Could you check a few things on this model? Use its own coordinates, in mm. Face numbers are marked on the shaded views. A direction names the side the tool comes from. Give positions to 0.01 mm unless a question says otherwise; leave off trailing zeros. Loops run counter-clockwise (first coordinate to the right, second up) from the corner with the lowest first, then second, coordinate; pieces in that order, holes last. Notation, with made-up numbers: M 75.5,-23 L 132.5,-23 A21 cw 132.5,1 Z; hole C 66,0.5 d9. An arc over 180 degrees is marked long. Use CSV: the item, a comma, the result in double quotes.
```python
from build123d import *

# Parameters (mm, degrees)
BASPROSKE_W         = 5
BASPROSKE_H         = 12.75
TOOTHCUT_DEPTH      = 19.711627401
TEETHCUTS_COUNT     = 15
TEETHCUTS_ANGLE     = 336
BORSKE_R            = 2.7
BORE_DEPTH          = 50.0049784
SKETCH3_R           = 2.7
BOSS_EXTRUDE2_DEPTH = 5
FILLET1_R           = 5


with BuildPart() as part:
    # BasProSke → Base-Revolve (revolve)
    with BuildSketch(Plane(origin=(0, 0, 0), x_dir=(1, 0, 0), z_dir=(0, 1, 0)), mode=Mode.PRIVATE) as base_revolve_sk:
        with Locations((2.5, 6.375)):
            Rectangle(BASPROSKE_W, BASPROSKE_H)
    revolve(base_revolve_sk.sketch.rotate(Axis((-10, 0, 0), (1, 0, 0)), 180), axis=Axis((-10, 0, 0), (1, 0, 0)))

    # TooCutSke → ToothCut (cut, through all)
    with BuildSketch(Plane(origin=(0, 0, 0), x_dir=(0, 0, -1), z_dir=(1, 0, 0))):
        with BuildLine():
            ThreePointArc((0.769645606, 9.34235097), (0, 9.374), (-0.769645606, 9.34235097))
            ThreePointArc((-0.769645606, 9.34235097), (-1.209019537, 11.113083179), (-2.315283452, 12.563849239))
            ThreePointArc((-2.315283452, 12.563849239), (0, 12.7754), (2.315283452, 12.563849239))
            ThreePointArc((2.315283452, 12.563849239), (1.209019537, 11.113083179), (0.769645606, 9.34235097))
        make_face()
    toothcut = extrude(amount=TOOTHCUT_DEPTH, mode=Mode.SUBTRACT)

    # TeethCuts: ToothCut ×15 about axis
    teethcuts_axis = Axis((-10, 0, 0), (1, 0, 0))
    for i in range(1, TEETHCUTS_COUNT):
        add(toothcut.rotate(teethcuts_axis, i * TEETHCUTS_ANGLE / (TEETHCUTS_COUNT - 1)), mode=Mode.SUBTRACT)

    # BorSke → Bore (cut, symmetric)
    with BuildSketch(Plane(origin=(0, 0, 0), x_dir=(0, 0, -1), z_dir=(1, 0, 0))):
        with Locations(Location((0, 0, 0), (0, 0, 180))):
            Circle(BORSKE_R)
    extrude(amount=BORE_DEPTH, both=True, mode=Mode.SUBTRACT)

    # Sketch3 → Boss-Extrude2 (add)
    with BuildSketch(Plane.ZY):
        with BuildLine():
            Line((-5.518933108, -11.493645085), (-4, -18.283482979))
            Line((-4, -18.283482979), (-4, -50))
            ThreePointArc((-4, -50), (0, -54), (4, -50))
            Line((4, -50), (4, -18.283482979))
            Line((4, -18.283482979), (5.518933108, -11.493645085))
            Line((5.518933108, -11.493645085), (2.695210989, -8.978179867))
            Line((2.695210989, -8.978179867), (-2.695210989, -8.978179867))
            Line((-2.695210989, -8.978179867), (-5.518933108, -11.493645085))
        make_face()
        with Locations((0, -50)):
            Circle(SKETCH3_R, mode=Mode.SUBTRACT)
    extrude(amount=-BOSS_EXTRUDE2_DEPTH)

    # Fillet1
    fillet1_edges = [part.edges().sort_by_distance(p)[0] for p in [
        (2.5, -18.283482979, -4),
        (2.5, -18.283482979, 4),
    ]]
    fillet(fillet1_edges, radius=FILLET1_R)


solid = part.part
```
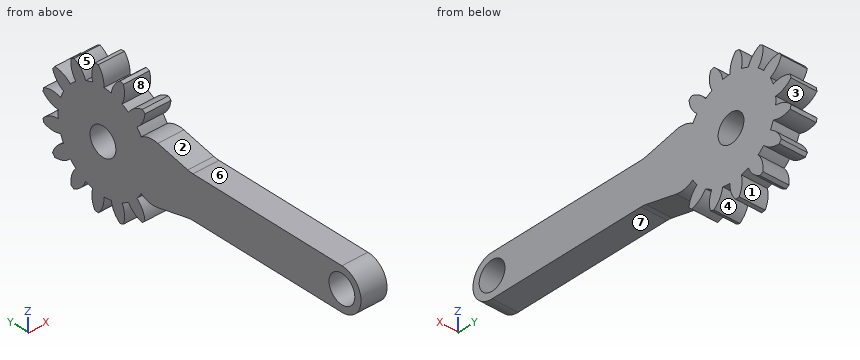
1. Which directions (+Z, -Z, +X, -X, +Y, -Y) give clear straight access to the entire face, cutting with the end or side of a thin tool? Please do the marked faces 4, 5, 6, 7 and 8.
Outcome:
face 4,"-Z, +X, -X"
face 5,"+Z, +X, -X"
face 6,"+Z, +X, -X, -Y"
face 7,"-Z, +X, -X, -Y"
face 8,"+X, -X"
2. I want a section at B-B, the plane x = 3.85. Give the number of separate pieces and of enclosed holes in the cut face, then the cut area to 3 significant figures.
Outcome:
separate pieces,"1"
enclosed holes,"2"
area,"686 mm2"
3. I want a section at C-C, the plane y = -34. List the corners of the cut face in (x, z) for me, then the cut area to 3 significant figures.
Outcome:
outline,"M 0,-4 L 5,-4 L 5,4 L 0,4 Z"
area,"40.0 mm2"
4. I want a section at A-A, the plane z = 0. List the corners of the cut face in (x, y) for me, then the cut area to 3 significant figures.
Outcome:
outline,"M 0,-54 L 5,-54 L 5,-52.7 L 0,-52.7 Z; M 0,-47.3 L 5,-47.3 L 5,-2.7 L 0,-2.7 Z; M 0,2.7 L 5,2.7 L 5,9.37 L 0,9.37 Z"
area,"263 mm2"
5. Please list where these lines run through material, in increasing order: line 1 (Y direction, x = 3.35, z = 0); line 2 (Z direction, x = 0.5, y = 9.5); line 3 (Z direction, x = 3.95, y = -27).
Outcome:
line 1,"-54 to -52.7, -47.3 to -2.7, 2.7 to 9.37"
line 2,"-7.75 to -5.45, -3.3 to -0.78, 0.78 to 3.3, 5.45 to 7.75"
line 3,"-4 to 4"
6. I'm going to push flat-ended pins straight in: pin 1 Ø1.5 at (x, y) = (2.5, -35.5) entering from +Z; pin 2 Ø4.5 at (y, z) = (-50, 0) entering from +X; pin 3 Ø12 at (y, z) = (-22.5, -7) entering from +X; pin 4 Ø1.5 at (x, z) = (4, -4) entering from -Y. Where does each tip first touch, or does it pass through?
Outcome:
pin 1,"z = 4"
pin 2,"through"
pin 3,"x = 5"
pin 4,"y = -52.33"
7. If we mould it in two halves opening along Y, with no side actions, what happens to the marked faces 1, 2 and 3? For each: +Y half, -Y half, draft (parallel to the pull), parting line (faces both ways), or undercut.
Outcome:
face 1,"undercut"
face 2,"-Y half"
face 3,"+Y half"
